from build123d import *

# Parameters (mm, degrees)
F1_DEPTH = 5.9
F2_DEPTH = 11.8
F3_DEPTH = 2.5


with BuildPart() as f1:
    # F0 (on Top) → F1 (new body)
    with BuildSketch(Plane.XY):
        with BuildLine():
            Line((3.475, 0.65), (3.475, 0))
            ThreePointArc((3.475, 0), (4.7730375063, 0.2208504846), (5.925, 0.8585484677))
            ThreePointArc((5.925, 0.8585484677), (6.5018486959, 1.426237912), (6.95, 2.1001712409))
            Line((6.95, 2.1001712409), (6.95, 5.7498287591))
            ThreePointArc((6.95, 5.7498287591), (5.5051689733, 7.2841723593), (3.475, 7.85))
            Line((3.475, 7.85), (3.475, 7.2))
            ThreePointArc((3.475, 7.2), (5.7907747084, 6.2407747084), (6.75, 3.925))
            ThreePointArc((6.75, 3.925), (5.7907747084, 1.6092252916), (3.475, 0.65))
        make_face()
        with BuildLine():
            Line((0, 5.7498287591), (0, 2.1001712409))
            ThreePointArc((0, 2.1001712409), (0.4481513041, 1.426237912), (1.025, 0.8585484677))
            ThreePointArc((1.025, 0.8585484677), (2.1769624937, 0.2208504846), (3.475, 0))
            Line((3.475, 0), (3.475, 0.65))
            ThreePointArc((3.475, 0.65), (0.2, 3.925), (3.475, 7.2))
            Line((3.475, 7.2), (3.475, 7.85))
            ThreePointArc((3.475, 7.85), (1.4448310267, 7.2841723593), (0, 5.7498287591))
        make_face()
        with BuildLine():
            Line((0, 2.1001712409), (0, 0))
            Line((0, 0), (1.025, 0))
            Line((1.025, 0), (1.025, 0.8585484677))
            ThreePointArc((1.025, 0.8585484677), (0.4481513041, 1.426237912), (0, 2.1001712409))
        make_face()
        with BuildLine():
            Line((1.025, 0.8585484677), (1.025, 0))
            Line((1.025, 0), (3.475, 0))
            ThreePointArc((3.475, 0), (2.1769624937, 0.2208504846), (1.025, 0.8585484677))
        make_face()
        with BuildLine():
            ThreePointArc((0, 5.7498287591), (-0.45, 3.925), (0, 2.1001712409))
            Line((0, 2.1001712409), (0, 5.7498287591))
        make_face()
        with BuildLine():
            Line((6.95, 5.7498287591), (6.95, 2.1001712409))
            ThreePointArc((6.95, 2.1001712409), (7.2858398025, 2.9852526935), (7.4, 3.925))
            ThreePointArc((7.4, 3.925), (7.2858398025, 4.8647473065), (6.95, 5.7498287591))
        make_face()
        with BuildLine():
            ThreePointArc((6.95, 2.1001712409), (6.5018486959, 1.426237912), (5.925, 0.8585484677))
            Line((5.925, 0.8585484677), (5.925, 0))
            Line((5.925, 0), (6.95, 0))
            Line((6.95, 0), (6.95, 1.44))
            Line((6.95, 1.44), (6.95, 1.5))
            Line((6.95, 1.5), (6.95, 2.1001712409))
        make_face()
        with BuildLine():
            ThreePointArc((5.925, 0.8585484677), (4.7730375063, 0.2208504846), (3.475, 0))
            Line((3.475, 0), (4.7, 0))
            Line((4.7, 0), (5.925, 0))
            Line((5.925, 0), (5.925, 0.8585484677))
        make_face()
        with BuildLine():
            Line((5.925, 0), (4.7, 0))
            add(Edge.make_bspline(
                [(4.7, 0), (5.2537494339, -0.3164176305), (5.6369397789, -0.7196032093), (5.925, -1.225)],
                knots=[0, 0, 0, 0, 1.7324116139, 1.7324116139, 1.7324116139, 1.7324116139], degree=3))
            Line((5.925, -1.225), (5.925, -0.079424061))
            Line((5.925, -0.079424061), (5.925, 0))
        make_face()
        with BuildLine():
            Line((6.95, 1.44), (6.95, 0))
            Line((6.95, 0), (9.8284865708, -0.079424061))
            add(Edge.make_bspline(
                [(6.95, 1.5), (7.7566024847, 0.7003984647), (8.7155010551, 0.2800084476), (9.8284865708, -0.079424061)],
                knots=[0, 0, 0, 0, 3.2833314336, 3.2833314336, 3.2833314336, 3.2833314336], degree=3))
            Line((6.95, 1.5), (6.95, 1.44))
        make_face()
    extrude(amount=-F1_DEPTH)

    # F0 (on Top) → F2 (join)
    with BuildSketch(Plane.XY):
        Polygon((8.29, -50.0240602729), (5.925, -50), (5.925, -52.0125), (5.925, -100), (8.29, -100), (8.29, -53.904), align=None)
        with BuildLine():
            add(Edge.make_bspline(
                [(5.925, -47.55), (5.2342489362, -48.7282052636), (4.4546769932, -49.3181198835), (3.475, -50)],
                knots=[0, 0, 0, 0, 3.4648232278, 3.4648232278, 3.4648232278, 3.4648232278], degree=3))
            Line((3.475, -50), (5.925, -50))
            Line((5.925, -50), (5.925, -47.55))
        make_face()
        Polygon((5.925, -50), (3.475, -50), (3.475, -100), (5.925, -100), (5.925, -52.0125), align=None)
        with BuildLine():
            Line((9.8284865708, -50.079424061), (9.8284865708, -50.0397120305))
            Line((9.8284865708, -50.0397120305), (8.29, -50.0240602729))
            Line((8.29, -50.0240602729), (8.29, -53.904))
            add(Edge.make_bspline(
                [(8.29, -53.904), (8.5714472143, -52.4050904341), (9.1968655396, -51.250747129), (10.207343012, -50.079424061)],
                knots=[0, 0, 0, 0, 4.2808358806, 4.2808358806, 4.2808358806, 4.2808358806], degree=3))
            Line((10.207343012, -50.079424061), (9.8284865708, -50.079424061))
        make_face()
        Polygon((9.8284865708, -25), (5.925, -25), (5.925, -26.9515), (5.925, -28.903), (5.925, -47.55), (5.925, -50), (8.29, -50), (9.8284865708, -50.0313035152), align=None)
        Polygon((12.1934865708, -0.079424061), (9.8284865708, -0.079424061), (9.8284865708, -25), (9.8284865708, -50.0313035152), (10.2417432854, -50.0397120305), (12.1934865708, -50.079424061), align=None)
        with BuildLine():
            Line((10.2417432854, -50.0397120305), (9.8284865708, -50.0313035152))
            Line((9.8284865708, -50.0313035152), (9.8284865708, -50.0397120305))
            Line((9.8284865708, -50.0397120305), (9.8284865708, -50.079424061))
            Line((9.8284865708, -50.079424061), (10.207343012, -50.079424061))
            add(Edge.make_bspline(
                [(10.207343012, -50.079424061), (10.2187605889, -50.0661890592), (10.230227327, -50.0529518896), (10.2417432854, -50.0397120305)],
                knots=[4.2808358806, 4.2808358806, 4.2808358806, 4.2808358806, 4.3292058583, 4.3292058583, 4.3292058583, 4.3292058583], degree=3))
        make_face()
        with BuildLine():
            Line((10.207343012, -50.079424061), (12.1934865708, -50.079424061))
            Line((12.1934865708, -50.079424061), (10.2417432854, -50.0397120305))
            add(Edge.make_bspline(
                [(10.207343012, -50.079424061), (10.2187605889, -50.0661890592), (10.230227327, -50.0529518896), (10.2417432854, -50.0397120305)],
                knots=[4.2808358806, 4.2808358806, 4.2808358806, 4.2808358806, 4.3292058583, 4.3292058583, 4.3292058583, 4.3292058583], degree=3))
        make_face()
        Polygon((9.8284865708, -50.0397120305), (9.8284865708, -50.0313035152), (8.29, -50), (8.29, -50.0240602729), align=None)
        Polygon((8.29, -50.0240602729), (8.29, -50), (5.925, -50), align=None)
        Polygon((6.95, 0), (5.925, 0), (5.925, -0.079424061), (5.925, -1.225), (5.925, -21.3844068348), (5.925, -22.55), (5.925, -22.9875), (5.925, -25), (9.8284865708, -25), (9.8284865708, -0.079424061), align=None)
    extrude(amount=-F2_DEPTH)

    # F0 (on Top) → F3 (join)
    with BuildSketch(Plane.XY):
        with BuildLine():
            Line((0, 7.85), (0, 5.7498287591))
            ThreePointArc((0, 5.7498287591), (1.4448310267, 7.2841723593), (3.475, 7.85))
            ThreePointArc((3.475, 7.85), (5.5051689733, 7.2841723593), (6.95, 5.7498287591))
            Line((6.95, 5.7498287591), (6.95, 17.9))
            Line((6.95, 17.9), (3.475, 17.9))
            Line((3.475, 17.9), (0, 17.9))
            Line((0, 17.9), (0, 7.85))
        make_face()
        with BuildLine():
            ThreePointArc((1.8276640256, 14.3833613398), (2.3042302705, 15.55900427), (3.475, 16.0474200003))
            ThreePointArc((3.475, 16.0474200003), (4.5253988967, 15.6691157612), (5.0933824344, 14.7079463483))
            Line((5.0933824344, 14.7079463483), (5.1024433757, 14.1442252627))
            Line((5.1024433757, 14.1442252627), (5.113982201, 13.4263440945))
            ThreePointArc((5.113982201, 13.4263440945), (5.1141409801, 13.4131724726), (5.1141939076, 13.4))
            ThreePointArc((5.1141939076, 13.4), (4.6340851277, 12.2409148723), (3.475, 11.7608060924))
            ThreePointArc((3.475, 11.7608060924), (2.2942628451, 12.2629791393), (1.8369719791, 13.4618131819))
            Line((1.8369719791, 13.4618131819), (1.8276640256, 14.3833613398))
        make_face(mode=Mode.SUBTRACT)
    extrude(amount=-F3_DEPTH)


solid = f1.part
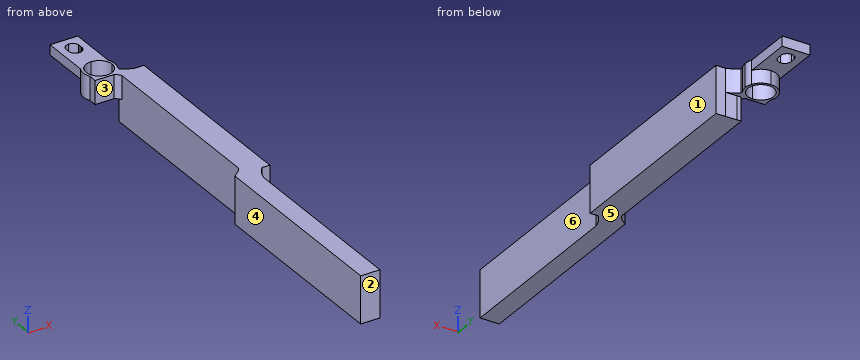
CAD build for the part. Positions are in the model's coordinates, mm. Face numbers are marked on the shaded views. A direction names the side the tool comes from. Coordinates: 2 decimals unless noted, no trailing zeros. Order: outer loops, then holes, each group sorted by start corner. A loop starts at its lowest first (then second) coordinate and runs counter-clockwise, first axis right, second up. Notation, with made-up numbers: (-7, 85.5) -> (51, 85.5) arc R21 ccw to (51, 98.5) -> close; hole circle Ø4 at (78, 31.25). An arc over 180 degrees is marked (long way). Answer in a Markdown table with one row per item.
1) Flat gauge pins, fed straight in: P1, Ø5, axis at x = 1.5, z = -4.5, coming from the -Y side; P2, Ø2.5, axis at y = 1.5, z = -3, coming from the -X side; P3, Ø1.1, axis at x = 6.5, z = -7.5, coming from the +Y side; P4, Ø7.5, axis at x = 3, y = 2.5, coming from the -Z side. Where does each tip first touch, or does it go through?
Check values:
| item | result |
|---|---|
| P1 | y = -100 |
| P2 | x = -0.27 |
| P3 | y = 0 |
| P4 | z = -5.9 |
2) Drill centre lines: line 1 (Z direction, x = 2, y = 8); line 2 (X direction, y = -79, z = -2.5) (3 decimals); line 3 (Y direction, x = 2.5, z = -5.75). Where is each one in solid material? Low to high.
Check values:
| item | result |
|---|---|
| line 1 | -2.5 to 0 |
| line 2 | 3.475 to 8.29 |
| line 3 | 0 to 0.8, 7.05 to 7.73 |
3) Band-saw the part on B-B (y = -60). List the corners of the cut face in (x, z) (3 decimals).
Check values:
| item | result |
|---|---|
| outline | (3.475, -11.8) -> (8.29, -11.8) -> (8.29, 0) -> (3.475, 0) -> close |
4) Which spindle directions (+Z, -Z, +X, -X, +Y, -Y) get a long thin tool onto all of the face, cutting with end or side? Do the marked faces 4, 5 and 6. Say none if no direction does.
Check values:
| item | result |
|---|---|
| face 4 | +Z, -Z, -X, -Y |
| face 5 | -Z, +X, -X, +Y, -Y |
| face 6 | +Z, -Z, +X, -Y |
5) Band-saw the part on A-A (y = -16.5). List the corners of the cut face in (x, z) (3 decimals), and give its area (3 significant figures).
Check values:
| item | result |
|---|---|
| outline | (5.925, -11.8) -> (12.193, -11.8) -> (12.193, 0) -> (5.925, 0) -> close |
| area | 74.0 mm2 |
6) Mould opens along Y. For the marked faces 1, 2 and 3 say: pulls with the +Y half, pulls with the -Y half, needs draft (parallel to the pull), parting line crosses it, or undercut.
Check values:
| item | result |
|---|---|
| face 1 | needs draft |
| face 2 | pulls with the -Y half |
| face 3 | undercut |
